Source: CAD feature listing. Evaluate the final solid. Frame: model axes, mm. Give positions to 0.01 mm unless a question says otherwise; leave off trailing zeros. Order: outer loops, then holes, each group sorted by start corner. A loop starts at its lowest first (then second) coordinate and runs counter-clockwise, first axis right, second up. Notation, with made-up numbers: M 55,83 L 77,83 A24 ccw 77,108 Z; hole C 2,-31 d8. An arc over 180 degrees is marked long. Answer in a Markdown table with one row per item. Add a question column.
(1) Mould query, pull axis X, two halves, no side actions, for faces 1 (the face through (-1, 0, 2)), 2 (the face through (50.773, 32.593, 1.014)), 3 (the face through (53.46, 0, 1)). Classes: pulls with the +X half, pulls with the -X half, needs draft (parallel to the pull), parting line crosses it, or undercut.
(2) Material intervals for line 1 along Y through (x, z) = (50.16, 0.85) (3 decimals), sorted ascending.
(3) Pin query (flat end, axial travel): P1, Ø4, axis at x = -5, y = 1, coming from the -Z side; P2, Ø2.5, axis at x = 50.16, y = 31.115, coming from the -Z side. Return the tip coordinate at first contact, or that it passes through.
(4) Section query A-A, the plane x = -50.28. Return loops of the section in (y, z) (3 decimals), plus the area to 3 significant figures.
Autodesk Fusion 360 part; units mm, degrees
sketch "Sketch1" plane through (0, 0, 0) normal (0, 0, 1) x (1, 0, 0)
  line L0 (53.46, -34.295) -> (-53.46, -34.295)
  line L1 (-53.46, -34.295) -> (-53.46, 34.295)
  line L2 (-53.46, 34.295) -> (53.46, 34.295)
  line L3 (53.46, 34.295) -> (53.46, -34.295)
  line L4 (53.46, -34.295) -> (-53.46, 34.295) construction
  line L5 (-53.46, -34.295) -> (53.46, 34.295) construction
  line L6 (-50.28, 31.115) -> (50.16, 31.115) construction
  line L7 (50.16, 31.115) -> (50.16, -31.115) construction
  line L8 (50.16, -31.115) -> (-50.28, -31.115) construction
  line L9 (-50.28, -31.115) -> (-50.28, 31.115) construction
  dimension "d1" = 106.92
  dimension "d2" = 68.59
  dimension "d5" = 3.18
  dimension "d6" = 3.18
  dimension "d7" = 100.44
  dimension "d8" = 62.23
extrude "Extrude1" add sketch "Sketch1" along normal blind 2
hole "Hole1" at (-50.28, 31.115, 0) at (-50.28, -31.115, 0) at (50.16, -31.115, 0) at (50.16, 31.115, 0) direction (0, 0, 1) diameter 3.2 end up to surface (2 mm away)
equation "d2 = 65.41 mm + 3.18 mm"
Values follow:
| question | item | result |
|---|---|---|
| 1 | face 1 | needs draft |
| 1 | face 2 | undercut |
| 1 | face 3 | pulls with the +X half |
| 2 | line 1 | y = -34.295 to -32.715, -29.515 to 29.515, 32.715 to 34.295 |
| 3 | P1 | stops at z = 0 |
| 3 | P2 | passes through |
| 4 | outline | M -34.295,0 L -32.715,0 L -32.715,2 L -34.295,2 Z; M -29.515,0 L 29.515,0 L 29.515,2 L -29.515,2 Z; M 32.715,0 L 34.295,0 L 34.295,2 L 32.715,2 Z |
| 4 | area | 124 mm² |
